Can you work these out from the model? Positions are in its coordinate system, mm. A direction names the side the tool comes from. Give positions to 0.01 mm unless a question says otherwise; leave off trailing zeros. Write each loop counter-clockwise with the first axis right and the second up, starting at its lowest first coordinate (ties: lowest second). Pieces come first, ordered by that corner, then holes.
1. Suppose I cut it at C-C (x = 0). Please give me the cut outline in (y, z), and give its area (3 significant figures).
2. Thinking about a two-plate mould opening in Y: for faces 5 (the cylindrical face through (0, -11, 27)), 6 (the cylindrical face through (-0.2, 21.5, 27.9)), 7 (the cylindrical face through (-8.998, 3.588, 27.014)), 8 (the flat face through (5, -2, 24)), which applies, pulls with the +Y half, pulls with the -Y half, needs draft (parallel to the pull), parting line crosses it, or undercut?
3. Suppose I cut it at A-A (z = 30.5). Please give me the cut outline in (x, y).
4. Suppose I cut it at D-D (y = 1). Please give me the cut outline in (x, z), and give its area (3 significant figures).
5. I'm going to push flat-ended pins straight in: pin 1 (2 mm diameter, centred on x = 0, y = 16, fed in from -Z); pin 2 (1 mm diameter, centred on x = -3.5, z = 30, fed in from +Y); pin 3 (1.2 mm diameter, centred on x = -3, z = 29, fed in from -Y). Where does each tip first touch, or does it pass through?
6. Suppose I cut it at B-B (z = 25). Please give me the cut outline in (x, y), and give its area (3 significant figures).
7. If I drill on probe 1 along Y at (x, z) = (0, 27.5); probe 2 along Y at (x, z) = (0, 24.7); probe 3 along Y at (x, z) = (-7, 24.65), over which ranges is the centre line in solid material (lowest first)?
8. On a 3-axis mill with a long thin cutter (end or side, diameter ignored), from which of +Z, -Z, +X, -X, +Y, -Y can I reach the whole of each face in a straight line? I mean faces 1 (the flat face through (-7, -6, 30)), 2 (the flat face through (-4, -9, 30)), 3 (the flat face through (0, 12, 31.6)), 4 (the cylindrical face through (5.002, 3.588, 27.014)). Say none if no direction works.
```python
from build123d import *

# Parameters (mm, degrees)
SKETCH_1_R          = 1.25
EXTRUDE_1_DEPTH     = 4
EXTRUDE_START       = -8
EXTRUDE_2_DEPTH     = 8
EXTRUDE_START_2     = -3
EXTRUDE_3_DEPTH     = 3
CUT_EXTRUDE_START   = -4
SKETCH_1_5_R        = 2
CUT_EXTRUDE_1_DEPTH = 6
SKETCH_4_W          = 20
SKETCH_4_H          = 17.5
CUT_EXTRUDE_2_DEPTH = 4
EXTRUDE_START_3     = -4
SKETCH_5_W          = 20
SKETCH_5_H          = 6
EXTRUDE_4_DEPTH     = 8
SKETCH_6_W          = 8
SKETCH_6_H          = 6
SKETCH_6_R          = 2
SKETCH_6_R_2        = 1.25
CUT_EXTRUDE_3_DEPTH = 4
SKETCH_6_3_R        = 1.25
CUT_EXTRUDE_4_DEPTH = 26.024987512
SKETCH_6_4_R        = 2
CUT_EXTRUDE_5_DEPTH = 6
SKETCH_7_R          = 0.9
CUT_EXTRUDE_6_DEPTH = 26.024987512
SKETCH_8_W          = 20
SKETCH_8_H          = 4.5
EXTRUDE_5_DEPTH     = 4
SKETCH_9_R          = 8.5
CUT_EXTRUDE_7_DEPTH = 1
SKETCH_10_R         = 2.55
CUT_EXTRUDE_8_DEPTH = 2.6
SKETCH_11_W         = 47.635441337
SKETCH_11_H         = 39.861258083
CUT_EXTRUDE_9_DEPTH = 30.769951293


with BuildPart() as part:
    # 草图1 → 凸台-拉伸1 (new, symmetric)
    with BuildSketch(Plane.XY):
        with BuildLine():
            Line((-10, 6), (-10, -6))
            Line((-10, -6), (10, -6))
            Line((10, -6), (10, 6))
            Line((10, 6), (6.480740698, 6))
            ThreePointArc((6.480740698, 6), (5.10105555, 4.70079179), (3.467802184, 3.739565217))
            ThreePointArc((3.467802184, 3.739565217), (0, -5.1), (-3.467802184, 3.739565217))
            ThreePointArc((-3.467802184, 3.739565217), (-5.10105555, 4.70079179), (-6.480740698, 6))
            Line((-6.480740698, 6), (-10, 6))
        make_face()
        with Locations((-7, 3.5)):
            Circle(SKETCH_1_R, mode=Mode.SUBTRACT)
        with Locations((7, 3.5)):
            Circle(SKETCH_1_R, mode=Mode.SUBTRACT)
    extrude(amount=EXTRUDE_1_DEPTH, both=True)

    # 草图2 → 凸台-拉伸2 (add)
    with BuildSketch(Plane(origin=(0, 0, -4), x_dir=(-1, 0, 0), z_dir=(0, 0, -1)).offset(EXTRUDE_START)):
        with BuildLine():
            Line((6.480740698, 6), (10, 6))
            Line((10, 6), (10, 11.5))
            ThreePointArc((10, 11.5), (0, 21.5), (-10, 11.5))
            Line((-10, 11.5), (-10, 6))
            Line((-10, 6), (-6.480740698, 6))
            ThreePointArc((-6.480740698, 6), (0, 20), (6.480740698, 6))
        make_face()
    extrude(amount=EXTRUDE_2_DEPTH)

    # 草图2<4> → 凸台-拉伸3 (add)
    with BuildSketch(Plane(origin=(0, 0, -4), x_dir=(-1, 0, 0), z_dir=(0, 0, -1)).offset(EXTRUDE_START_2)):
        with BuildLine():
            Line((-6.480740698, 6), (6.480740698, 6))
            ThreePointArc((6.480740698, 6), (7.979232292, 8.570520177), (8.5, 11.5))
            ThreePointArc((8.5, 11.5), (-2.929479823, 19.479232292), (-6.480740698, 6))
        make_face()
    extrude(amount=EXTRUDE_3_DEPTH)

    # 草图1<5> → 切除-拉伸1 (cut)
    with BuildSketch(Plane.XY.offset(CUT_EXTRUDE_START)):
        with Locations((-7, 3.5)):
            Circle(SKETCH_1_5_R)
        with Locations((7, 3.5)):
            Circle(SKETCH_1_5_R)
    extrude(amount=CUT_EXTRUDE_1_DEPTH, mode=Mode.SUBTRACT)

    # 草图4 → 切除-拉伸2 (cut)
    with BuildSketch(Plane(origin=(0, 0, -4), x_dir=(-1, 0, 0), z_dir=(0, 0, -1))):
        with Locations((0, 2.75)):
            Rectangle(SKETCH_4_W, SKETCH_4_H)
    extrude(amount=-CUT_EXTRUDE_2_DEPTH, mode=Mode.SUBTRACT)

    # 草图5 → 凸台-拉伸4 (add)
    with BuildSketch(Plane(origin=(0, 0, 0), x_dir=(-1, 0, 0), z_dir=(0, 0, -1)).offset(EXTRUDE_START_3)):
        with Locations((0, -9)):
            Rectangle(SKETCH_5_W, SKETCH_5_H)
    extrude(amount=EXTRUDE_4_DEPTH)

    # 草图6 → 切除-拉伸3 (cut)
    # profile 1 of 3: a face of its own
    with BuildSketch(Plane(origin=(0, 0, -4), x_dir=(-1, 0, 0), z_dir=(0, 0, -1))):
        with Locations((0, -9)):
            Rectangle(SKETCH_6_W, SKETCH_6_H)
        with Locations((0, -9)):
            Circle(SKETCH_6_R, mode=Mode.SUBTRACT)
    # profile 2 of 3: a face of its own
    with BuildSketch(Plane(origin=(0, 0, -4), x_dir=(-1, 0, 0), z_dir=(0, 0, -1))):
        with Locations((0, -9)):
            Circle(SKETCH_6_R)
        with Locations((0, -9)):
            Circle(SKETCH_6_R_2, mode=Mode.SUBTRACT)
    # profile 3 of 3: a face of its own
    with BuildSketch(Plane(origin=(0, 0, -4), x_dir=(-1, 0, 0), z_dir=(0, 0, -1))):
        with Locations((0, -9)):
            Circle(SKETCH_6_R_2)
    extrude(amount=-CUT_EXTRUDE_3_DEPTH, mode=Mode.SUBTRACT)

    # 草图6<3> → 切除-拉伸4 (cut, through all)
    with BuildSketch(Plane(origin=(0, 0, -4), x_dir=(-1, 0, 0), z_dir=(0, 0, -1))):
        with Locations((0, -9)):
            Circle(SKETCH_6_3_R)
    extrude(amount=-CUT_EXTRUDE_4_DEPTH, mode=Mode.SUBTRACT)

    # 草图6<4> → 切除-拉伸5 (cut)
    with BuildSketch(Plane(origin=(0, 0, -4), x_dir=(-1, 0, 0), z_dir=(0, 0, -1))):
        with Locations(Location((0, -9, 0), (0, 0, 180))):
            Circle(SKETCH_6_4_R)
    extrude(amount=-CUT_EXTRUDE_5_DEPTH, mode=Mode.SUBTRACT)

    # 草图7 → 切除-拉伸6 (cut, through all)
    with BuildSketch(Plane(origin=(0, 0, -4), x_dir=(-1, 0, 0), z_dir=(0, 0, -1))):
        with Locations((7, -9)):
            Circle(SKETCH_7_R)
        with Locations((-7, -9)):
            Circle(SKETCH_7_R)
        with Locations((0, 16)):
            Circle(SKETCH_7_R)
    extrude(amount=-CUT_EXTRUDE_6_DEPTH, mode=Mode.SUBTRACT)

    # 草图8 → 凸台-拉伸5 (add)
    with BuildSketch(Plane(origin=(0, 0, 0), x_dir=(-1, 0, 0), z_dir=(0, 0, -1))):
        with Locations((0, 9.25)):
            Rectangle(SKETCH_8_W, SKETCH_8_H)
    extrude(amount=EXTRUDE_5_DEPTH)

    # 草图9 → 切除-拉伸7 (cut)
    with BuildSketch(Plane.XY):
        with Locations((0, 11.5)):
            Circle(SKETCH_9_R)
    extrude(amount=-CUT_EXTRUDE_7_DEPTH, mode=Mode.SUBTRACT)

    # 草图10 → 切除-拉伸8 (cut)
    with BuildSketch(Plane.XY.offset(-1)):
        with Locations((0, 11.5)):
            Circle(SKETCH_10_R)
    extrude(amount=-CUT_EXTRUDE_8_DEPTH, mode=Mode.SUBTRACT)


with BuildPart() as body_2:
    # 镜向1: mirrored copy
    add(part.part.mirror(Plane.XY.offset(14)))


with BuildPart() as part_1:
    add(part.part)

    # 草图11 → 切除-拉伸9 (cut, through all)
    with BuildSketch(Plane.XY.offset(14)):
        with Locations((-3.268127992, 5.220412363)):
            Rectangle(SKETCH_11_W, SKETCH_11_H)
    extrude(amount=-CUT_EXTRUDE_9_DEPTH, mode=Mode.SUBTRACT)


solid = body_2.part
```
Checks:
1. outline: (-12, 24) - (-10.25, 24) - (-10.25, 26) - (-11, 26) - (-11, 28) - (-12, 28) - close; (-7.75, 24) - (-5.1, 24) - (-5.1, 28) - (-7, 28) - (-7, 26) - (-7.75, 26) - close; (7, 29) - (8.95, 29) - (8.95, 31.6) - (14.05, 31.6) - (14.05, 29) - (15.1, 29) - (15.1, 32) - (7, 32) - close; (16.9, 29) - (20, 29) - (20, 24) - (21.5, 24) - (21.5, 32) - (16.9, 32) - close
1. area: 46.9 mm2
2. face 5: undercut
2. face 6: pulls with the +Y half
2. face 7: undercut
2. face 8: needs draft
3. outline: (-10, -12) - (-4, -12) - (-4, -6) - (-10, -6) - close; (-10, 7) - (10, 7) - (10, 11.5) arc R10 ccw to (-10, 11.5) - close; (4, -12) - (10, -12) - (10, -6) - (4, -6) - close; hole circle Ø1.8 at (-7, -9); hole circle Ø5.1 at (0, 11.5); hole circle Ø1.8 at (0, 16); hole circle Ø1.8 at (7, -9)
4. outline: (-10, 24) - (-5, 24) - (-5, 28) - (-10, 28) - close; (5, 24) - (10, 24) - (10, 28) - (5, 28) - close
4. area: 40.0 mm2
5. pin 1: stops at z = 29
5. pin 2: stops at y = 21.04
5. pin 3: stops at y = 7
6. outline: (-10, -12) - (10, -12) - (10, 11.5) arc R10 ccw to (-10, 11.5) - close; hole circle Ø2.5 at (-7, 3.5); hole circle Ø1.8 at (-7, -9); hole (-3.47, 3.74) arc R5.1 ccw (long way) to (3.47, 3.74) arc R8.5 ccw (long way) to start; hole circle Ø2.5 at (0, -9); hole circle Ø2.5 at (7, 3.5); hole circle Ø1.8 at (7, -9)
6. area: 309 mm2
7. probe 1: y = -12 to -11, -7 to -5.1, 20 to 21.5
7. probe 2: y = -12 to -10.25, -7.75 to -5.1, 20 to 21.5
7. probe 3: y = -12 to -9.9, -8.1 to 2.25, 4.75 to 6.68, 16.32 to 18.64
8. face 1: +Z, +X, -X
8. face 2: +Z, -Y
8. face 3: -Z
8. face 4: +Z
